from build123d import *

# Parameters (mm, degrees)
F_4_0_4_DIAMETER_HOLE1_D = 4


with BuildPart() as part:
    # Sketch1 → Revolve1 (revolve)
    with BuildSketch(Plane(origin=(0, 0, 0), x_dir=(0, 0, -1), z_dir=(1, 0, 0)), mode=Mode.PRIVATE) as revolve1_sk:
        Polygon((0, 0), (0, 3), (-7, 3), (-7, 3.175), (-19.5, 3.175), (-19.5, 4), (-27.5, 4), (-27.5, 5), (-36.5, 6), (-74.5, 6), (-83.5, 5), (-83.5, 4), (-92.5, 4), (-92.5, 3), (-117, 3), (-117, 2.95), (-127, 2.95), (-127, 0), align=None)
    revolve(revolve1_sk.sketch.rotate(Axis((0, 0, 0), (0, 0, 1)), 90), axis=Axis((0, 0, 0), (0, 0, 1)))

    # Ø4.0 (4) Diameter Hole1 (through all)
    with Locations(Plane(origin=(0, 0, 0), x_dir=(-1, 0, 0), z_dir=(0, 0, -1))):
        with Locations((0, 0)):
            Hole(F_4_0_4_DIAMETER_HOLE1_D / 2)


solid = part.part
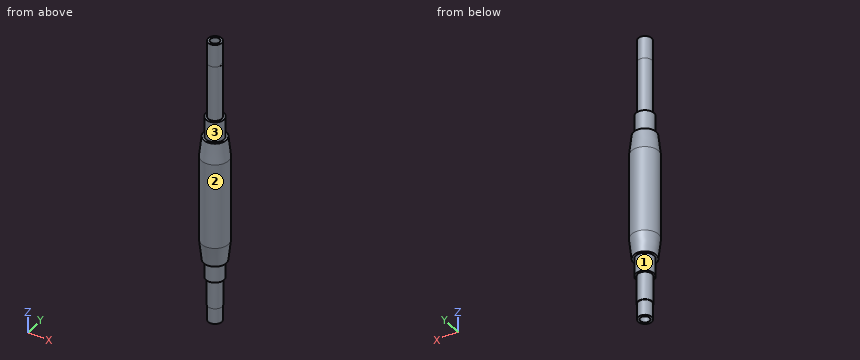
Geometry: final body of the model. Coordinates: model frame, mm. Face numbers are marked on the shaded views. A direction names the side the tool comes from. Round coordinates to 2 decimals unless told otherwise and drop trailing zeros. Loops run counter-clockwise (first coordinate to the right, second up) from the corner with the lowest first, then second, coordinate; pieces in that order, holes last.
Q1. Section A-A on z = 15. Return loops of the section in (x, y) (3 decimals), plus the area to 3 significant figures.
Q2. Section B-B on z = 94. Return loops of the section in (x, y).
Q3. Pin query (flat end, axial travel): P1, Ø1.5, axis at y = -3.5, z = 18.5, coming from the +X side; P2, Ø1.5, axis at x = -3, y = 4, coming from the +Z side; P3, Ø3, axis at x = -4, z = 82, coming from the +Y side. Return the tip coordinate at first contact, or that it passes through.
Q4. Access query for the marked faces 1, 2 and 3. Directions: +Z, -Z, +X, -X, +Y, -Y. A direction counts if a zero-diameter tool reaches every point of the face in a straight line with its end or side. Return the directions, or none.
Q5. Material intervals for L1, parallel to Y at x = 0, z = 26; L2, parallel to Y at x = 0, z = 74; L3, parallel to X at y = 1, z = 110, sorted ascending.
Evaluation:
1. outline: circle Ø6.35 at (0, 0); hole circle Ø4 at (0, 0)
1. area: 19.1 mm2
2. outline: circle Ø6 at (0, 0); hole circle Ø4 at (0, 0)
3. P1: stops at x = 1.59
3. P2: stops at z = 83.5
3. P3: stops at y = 4.54
4. face 1: -Z
4. face 2: +Z, -Z
4. face 3: +Z
5. L1: y = -4 to -2, 2 to 4
5. L2: y = -6 to -2, 2 to 6
5. L3: x = -2.83 to -1.73, 1.73 to 2.83
